Answer from the drawing. Dimensions are ordinates in mm from the lowest x, y and z of the part. A direction names the side the tool comes from. Give positions to 0.01 mm unless a question says otherwise; leave off trailing zeros. Order: outer loops, then holes, each group sorted by start corner. A loop starts at its lowest first (then second) coordinate and runs counter-clockwise, first axis right, second up.
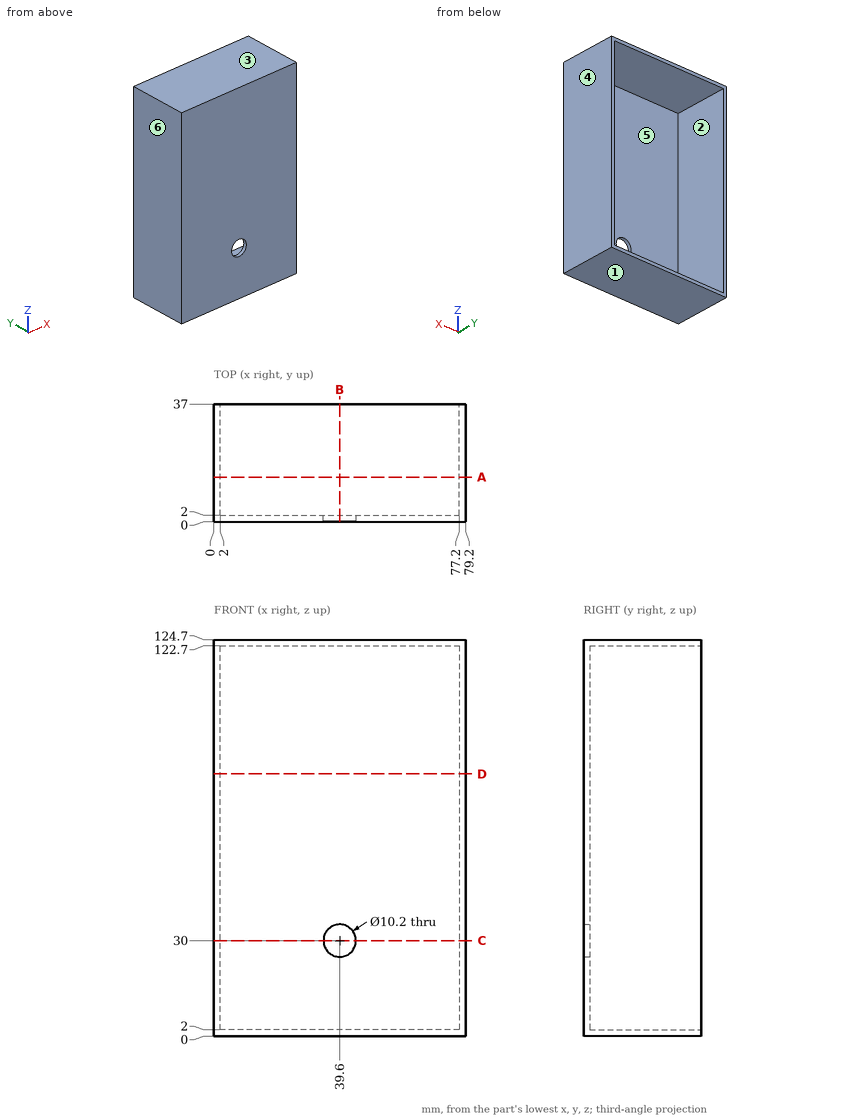
1) Given pin 1 (10.5 mm diameter, centred on y = 19, z = 71.5, fed in from -X); pin 2 (4 mm diameter, centred on x = 59, z = 99.5, fed in from +Y), each flat-ended and moving along its own axis, determine where each tip first touches the part or whether it passes through.
Final values:
pin 1: stops at x = 0
pin 2: stops at y = 2
2) A tool of negligible diameter and unlimited length cuts with its end or side. For the marked faces 1 and 2, from which of +Z, -Z, +X, -X, +Y, -Y can it reach the whole face along a straight path? Write none if from no direction.
Final values:
face 1: -Z, +X, -X, +Y, -Y
face 2: +Y
3) The part is cut by section C-C on z = 30. Determine the outline of the cut face in (x, y).
Final values:
outline: (0, 0) - (34.5, 0) - (34.5, 2) - (2, 2) - (2, 37) - (0, 37) - close; (44.7, 0) - (79.2, 0) - (79.2, 37) - (77.2, 37) - (77.2, 2) - (44.7, 2) - close
4) The part is cut by section D-D on z = 82.5. Determine the outline of the cut face in (x, y).
Final values:
outline: (0, 0) - (79.2, 0) - (79.2, 37) - (77.2, 37) - (77.2, 2) - (2, 2) - (2, 37) - (0, 37) - close
5) The part is cut by section A-A on y = 14. Determine the outline of the cut face in (x, z), and give its area (3 significant figures).
Final values:
outline: (0, 0) - (79.2, 0) - (79.2, 124.7) - (0, 124.7) - close; hole (2, 2) - (77.2, 2) - (77.2, 122.7) - (2, 122.7) - close
area: 800 mm2
6) The part is cut by section B-B on x = 39.6. Determine the outline of the cut face in (y, z).
Final values:
outline: (0, 0) - (37, 0) - (37, 2) - (2, 2) - (2, 24.9) - (0, 24.9) - close; (0, 35.1) - (2, 35.1) - (2, 122.7) - (37, 122.7) - (37, 124.7) - (0, 124.7) - close
7) For a pull along X with two mould halves and no side action, classify the marked faces 3, 4, 5 and 6 as released by +X, released by -X, zero draft, split by the parting line, or undercut.
Final values:
face 3: zero draft
face 4: released by +X
face 5: undercut
face 6: released by -X
8) Consider L1, parallel to X at y = 30.5, z = 67; L2, parallel to Z at x = 25, y = 7; L3, parallel to Y at x = 51.5, z = 50. Determine where each line is inside the solid, lowest interval first.
Final values:
L1: x = 0 to 2, 77.2 to 79.2
L2: z = 0 to 2, 122.7 to 124.7
L3: y = 0 to 2
